Source: CAD feature listing. Evaluate the final solid. Frame: model axes, mm. A direction names the side the tool comes from. Give positions to 0.01 mm unless a question says otherwise; leave off trailing zeros. Order: outer loops, then holes, each group sorted by start corner. A loop starts at its lowest first (then second) coordinate and runs counter-clockwise, first axis right, second up.
1) Section A-A, the plane x = 8. Return loops of the section in (y, z).
2) Section B-B, the plane z = 0. Return loops of the section in (x, y), plus the area to 4 significant figures.
3) Section C-C, the plane x = -12. Return loops of the section in (y, z).
4) First-contact query: P1, Ø1.6, axis at x = -12, y = 3, coming from the -Z side; P2, Ø1.5, axis at y = 20.5, z = -11.5, coming from the -X side; P3, Ø2, axis at x = -5, y = 3, coming from the -Z side; P4, Ø0.6, axis at x = -11.5, y = 3.5, coming from the +Z side. Flat tips, straight axial feed; report the tip coordinate or a pass-through.
5) Access query for faces 4 (the face through (-0.5, 10.7, 0.1)), 5 (the face through (-11, 4, -1)). Directions: +Z, -Z, +X, -X, +Y, -Y. A direction counts if a zero-diameter tool reaches every point of the face in a straight line with its end or side. Return the directions, or none.
6) Draft query along Y for faces 1 (the face through (4, 6.5, 0)), 2 (the face through (0, 0, 0)), 3 (the face through (-10.49, 13.32, 0.46)). Return one class per face: released by +Y, released by -Y, zero draft, split by the parting line, or undercut.
7) Section D-D, the plane y = 23.25. Return loops of the section in (x, z).
8) Material intervals for line 1 (Y direction, x = 0, z = -6.25); line 2 (Y direction, x = -3.25, z = 12); line 3 (X direction, y = 8.5, z = -1), sorted ascending.
Autodesk Inventor part; units mm, degrees
ref_plane "作業平面1" through (0, 6.5, 0) normal (0, 1, 0) x (1, 0, 0)
ref_plane "YZ Plane" through (0, 0, 0) normal (1, 0, 0) x (0, 1, 0)
ref_plane "XZ Plane" through (0, 0, 0) normal (0, 1, 0) x (-1, 0, 0)
sketch "スケッチ1" plane through (0, 0, 0) normal (0, 1, 0) x (-1, 0, 0)
  circle A0 centre (0, 0) radius 15
  dimension "d0" = 30
extrude "押し出し1" add sketch "スケッチ1" along normal blind 1
sketch "スケッチ2" plane through (0, 1, 0) normal (0, 1, 0) x (1, 0, 0)
  circle A0 centre (0, 0) radius 10.5
  dimension "d3" = 21
extrude "押し出し2" add sketch "スケッチ2" along normal blind 25
ref_plane "作業平面1" through (0, 6.5, 0) normal (0, 1, 0) x (1, 0, 0)
sketch "スケッチ4" plane through (0, 6.5, 0) normal (0, 1, 0) x (1, 0, 0)
  circle A0 centre (0, 0) radius 10.5
  circle A1 centre (79.5, 0) radius 80
  point P0 (0.1918, 10.4982)
  point P1 (0.1918, -10.4982)
  dimension "d9" = 79.5
  dimension "d10" = 160
extrude "押し出し3" cut sketch "スケッチ4" along normal blind 8.5 contours A0 A1 picked at (3.218, 0)
sketch "スケッチ5" plane through (0, 1, 0) normal (0, 1, 0) x (1, 0, 0)
  line L0 (-15, 1) -> (-8.9813, 1)
  line L1 (-8.9813, 1) -> (-8.9813, -1)
  line L2 (-8.9813, -1) -> (-15, -1)
  line L3 (-15, -1) -> (-15, 1)
  circle A0 centre (0, 0) radius 15
  circle A1 centre (0, 0) radius 12.5
  point P0 (-15, 0)
  point P1 (-14.9666, 1)
  point P2 (-14.9666, -1)
  point P3 (-12.4599, 1)
  point P4 (-12.4599, -1)
  dimension "d11" = 2
  dimension "d14" = 25
extrude "押し出し4" add sketch "スケッチ5" along normal blind 5.5 contours L0 L1 L2 A1 picked at (-10.1527, -0.1112)
properties part number "ギア軸_中心"
From the geometry:
1. outline: (0, -12.69) - (1, -12.69) - (1, -6.8) - (6.5, -6.8) - (6.5, 6.8) - (1, 6.8) - (1, 12.69) - (0, 12.69) - close; (15, -6.8) - (26, -6.8) - (26, 6.8) - (15, 6.8) - close
2. outline: (-15, 0) - (15, 0) - (15, 1) - (10.5, 1) - (10.5, 6.5) - (-0.5, 6.5) - (-0.5, 15) - (10.5, 15) - (10.5, 26) - (-10.5, 26) - (-10.5, 6.5) - (-12.5, 6.5) - (-12.5, 1) - (-15, 1) - close
2. area: 472.5 mm2
3. outline: (0, -9) - (1, -9) - (1, -1) - (6.5, -1) - (6.5, 1) - (1, 1) - (1, 9) - (0, 9) - close
4. P1: stops at z = -1
4. P2: passes through
4. P3: stops at z = -9.71
4. P4: stops at z = 1
5. face 4: +X
5. face 5: -Z, -X, +Y
6. face 1: undercut
6. face 2: released by -Y
6. face 3: zero draft
7. outline: circle Ø21 at (0, 0)
8. line 1: y = 0 to 6.5, 15 to 26
8. line 2: y = 0 to 1
8. line 3: x = -10.45 to -0.49
